Could you check a few things on this model? Use its own coordinates, in mm. Face numbers are marked on the shaded views. Round coordinates to 2 decimals unless told otherwise and drop trailing zeros. Order: outer loops, then holes, each group sorted by start corner. A loop starts at its lowest first (then second) coordinate and runs counter-clockwise, first axis right, second up. Notation, with made-up numbers: (36.25, 58) -> (53.25, 58) arc R8 ccw to (53.25, 71) -> close; hole circle Ø5 at (-4, 67.25). An arc over 180 degrees is marked (long way). One line per question, with ' | ' between items.
```python
from build123d import *

# Parameters (mm, degrees)
SKETCH062_R  = 1.25
PAD029_DEPTH = 1.8
SKETCH063_R  = 1.25
PAD031_DEPTH = 3
FILLET003_R  = 2


with BuildPart() as part:
    # Sketch062 → Pad029 (new body, symmetric)
    with BuildSketch(Plane.YZ.offset(-41.1)):
        with BuildLine():
            Line((96.000005, 10.999996), (100.999998, 10.999996))
            Line((100.999998, 10.999996), (100.999998, 27))
            Line((100.999998, 27), (92.999998, 17.465971))
            Line((92.999998, 14), (92.999998, 17.465971))
            ThreePointArc((92.999998, 14), (93.878624, 11.87862), (96.000005, 10.999996))
        make_face()
        with Locations((97, 15)):
            Circle(SKETCH062_R, mode=Mode.SUBTRACT)
    extrude(amount=PAD029_DEPTH, both=True)

    # Sketch063 (on Face8 of Clone025) → Pad031 (new body)
    with BuildSketch(Plane.YZ.offset(-39.3)):
        with BuildLine():
            Line((100.999998, 27), (92.999998, 17.465971))
            Line((92.999998, 17.465971), (92.999998, 14))
            ThreePointArc((92.999998, 14), (93.87868, 11.878676), (96.000005, 10.999996))
            Line((96.000005, 10.999996), (100.999998, 10.999996))
            Line((100.999998, 10.999996), (100.999998, 27))
        make_face()
        with Locations((97, 15)):
            Circle(SKETCH063_R, mode=Mode.SUBTRACT)
    extrude(amount=PAD031_DEPTH)

    # Fillet003
    fillet003_edges = [part.edges().sort_by_distance(p)[0] for p in [
        (-36.3, 98.500001, 10.999996),
        (-36.3, 93.87868, 11.878676),
        (-36.3, 92.999998, 15.732986),
        (-36.3, 96.999998, 22.232986),
    ]]
    fillet(fillet003_edges, radius=FILLET003_R)


solid = part.part
```
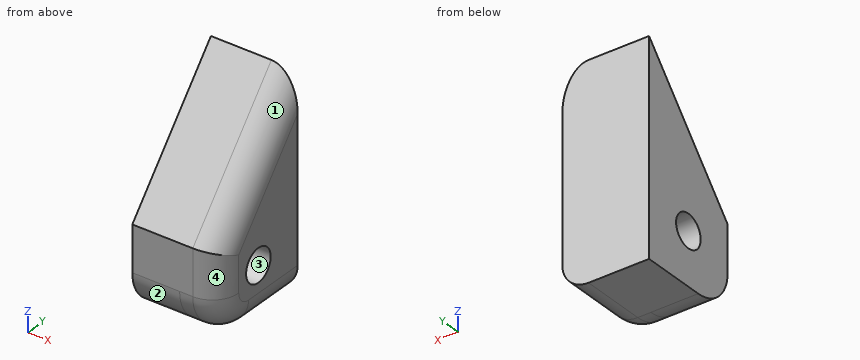
1. I'm going to push flat-ended pins straight in: pin 1 (4 mm diameter, centred on y = 97, z = 15, fed in from +X); pin 2 (1.5 mm diameter, centred on x = -38, y = 96, fed in from +Z); pin 3 (1 mm diameter, centred on x = -39, z = 24, fed in from -Y). Where does each tip first touch, or does it pass through?
From the geometry:
pin 1: stops at x = -36.3 | pin 2: stops at z = 21.91 | pin 3: stops at y = 98.06
2. I want a section at A-A on z = 15. List the corners of the cut face in (x, y) for me.
From the geometry:
outline: (-42.9, 93) -> (-38.3, 93) arc R2 ccw to (-36.3, 95) -> (-36.3, 95.75) -> (-42.9, 95.75) -> close; (-42.9, 98.25) -> (-36.3, 98.25) -> (-36.3, 101) -> (-42.9, 101) -> close
3. If we mould it in two halves opening along Z, with no side actions, what happens to the marked faces 1, 2, 3 and 4? For each: pulls with the +Z half, pulls with the -Z half, needs draft (parallel to the pull), parting line crosses it, or undercut.
From the geometry:
face 1: pulls with the +Z half | face 2: pulls with the -Z half | face 3: undercut | face 4: needs draft
4. I need wall thicknesses on probe 1 along Y at (x, z) = (-39.5, 14.5); probe 2 along Z at (x, y) = (-40.25, 97); probe 3 along Y at (x, z) = (-41.5, 25.5). Which ranges of each line are inside material? Lowest first, please.
From the geometry:
probe 1: y = 93 to 95.85, 98.15 to 101 | probe 2: z = 11 to 13.75, 16.25 to 22.23 | probe 3: y = 99.74 to 101
5. I want a section at B-B on x = -40.5. List the corners of the cut face in (y, z) for me, and give its area (3 significant figures).
From the geometry:
outline: (93, 14) arc R3 ccw to (96, 11) -> (101, 11) -> (101, 27) -> (93, 17.47) -> close; hole circle Ø2.5 at (97, 15) | area: 83.0 mm²
